Could you check a few things on this model? Use its own coordinates, in mm. A direction names the side the tool comes from. Coordinates: 2 decimals unless noted, no trailing zeros. Order: outer loops, then holes, each group sorted by start corner. A loop starts at its lowest first (then second) coordinate and runs counter-clockwise, first axis right, second up. Notation, with made-up numbers: (88, -19) -> (143, -19) arc R16 cw to (143, -10) -> close; hole circle Ø3 at (45, -25.5). An arc over 180 degrees is marked (long way). Use a Markdown table: item, result. Add a question column.
1) If we section it at C-C (y = 21): Write out the boundary of the cut face in (x, z), plus the area to 3 significant figures.
2) Will these pins go through, and if not, where does the flat tip stop? pin 1 Ø13 at (x, y) = (41.5, 57.5) entering from +Z; pin 2 Ø5 at (x, y) = (41.5, 57.5) entering from +Z; pin 3 Ø3 at (x, y) = (-41.5, 57.5) entering from +Z.
3) If we section it at B-B (y = -14.5): Write out the boundary of the cut face in (x, z).
4) If I drill on L1, parallel to Y at x = -41.5, z = 7.7; L2, parallel to X at y = 22, z = 1.75; L3, parallel to X at y = 32, z = 4, over which ranges is the centre line in solid material (lowest first)? Write a range as [from, to].
5) If we section it at A-A (x = 21.5): Write out the boundary of the cut face in (y, z).
6) Which directions (+Z, -Z, +X, -X, +Y, -Y) give clear straight access to the entire face, cutting with the end or side of a thin tool? Please do faces 5 (the flat face through (21.904, -4.523, 5.07)), 6 (the flat face through (-65, -2, 5)), 7 (the cylindrical face through (37.5, -28.5, 8)).
7) Thinking about a two-plate mould opening in Y: for faces 1 (the flat face through (-30.24, 46.57, 5.07)), 2 (the flat face through (14, 2, 0)), 3 (the cylindrical face through (-5.62, -26.266, 5.07)), 4 (the flat face through (-1, 120, 5)), which applies, +Y half, -Y half, draft (parallel to the pull), parting line (faces both ways), or undercut?
```python
from build123d import *

# Parameters (mm, degrees)
SKETCH008_W          = 130
SKETCH008_H          = 240
PAD005_DEPTH         = 10
SKETCH009_R          = 2
POCKET003_DEPTH      = 10.001
POCKET003_DEPTH_BACK = 0.001
SKETCH010_R          = 5
POCKET004_DEPTH      = 4
POCKET005_DEPTH      = 10.001
POCKET005_DEPTH_BACK = 0.001


with BuildPart() as part:
    # Sketch008 → Pad005 (new body)
    with BuildSketch(Plane.XY):
        Rectangle(SKETCH008_W, SKETCH008_H)
    extrude(amount=PAD005_DEPTH)

    # Sketch009 (on Face5 of Pad005) → Pocket003 (cut, two sides)
    with BuildSketch(Plane(origin=(0, 0, 0), x_dir=(1, 0, 0), z_dir=(0, 0, -1))) as pocket003_sk:
        with Locations((-41.5, -57.5)):
            Circle(SKETCH009_R)
        with Locations((-41.5, 25.5)):
            Circle(SKETCH009_R)
        with Locations((41.5, 25.5)):
            Circle(SKETCH009_R)
        with Locations((41.5, -57.5)):
            Circle(SKETCH009_R)
    extrude(amount=-POCKET003_DEPTH, mode=Mode.SUBTRACT)
    extrude(pocket003_sk.sketch, amount=POCKET003_DEPTH_BACK, mode=Mode.SUBTRACT)

    # Sketch010 (on Face5 of Pocket003) → Pocket004 (cut)
    with BuildSketch(Plane.XY.offset(10)):
        with Locations((-41.5, 57.5)):
            Circle(SKETCH010_R)
        with Locations((41.5, 57.5)):
            Circle(SKETCH010_R)
        with Locations((-41.5, -25.5)):
            Circle(SKETCH010_R)
        with Locations((41.5, -25.5)):
            Circle(SKETCH010_R)
    extrude(amount=-POCKET004_DEPTH, mode=Mode.SUBTRACT)

    # Sketch011 (on Face5 of Pocket004) → Pocket005 (cut, two sides)
    with BuildSketch(Plane.XY.offset(10)) as pocket005_sk:
        with BuildLine():
            ThreePointArc((-33.328427, -11.671573), (-33.328427, -17.328427), (-27.671573, -17.328427))
            Line((-27.671573, -17.328427), (33.328427, 43.671573))
            ThreePointArc((33.328427, 43.671573), (33.328427, 49.328427), (27.671573, 49.328427))
            Line((27.671573, 49.328427), (-33.328427, -11.671573))
        make_face()
        with BuildLine():
            ThreePointArc((-42.328427, -2.286797), (-42.328427, -7.943651), (-36.671573, -7.943651))
            Line((-36.671573, -7.943651), (23.943651, 52.671573))
            ThreePointArc((23.943651, 52.671573), (23.943651, 58.328427), (18.286797, 58.328427))
            Line((18.286797, 58.328427), (-42.328427, -2.286797))
        make_face()
        with BuildLine():
            ThreePointArc((-42.328427, 16.09798), (-42.328427, 10.441125), (-36.671573, 10.441125))
            Line((-36.671573, 10.441125), (5.558875, 52.671573))
            ThreePointArc((5.558875, 52.671573), (5.558875, 58.328427), (-0.09798, 58.328427))
            Line((-0.09798, 58.328427), (-42.328427, 16.09798))
        make_face()
        with BuildLine():
            ThreePointArc((-42.328427, 34.482756), (-42.328427, 28.825902), (-36.671573, 28.825902))
            Line((-36.671573, 28.825902), (-12.825902, 52.671573))
            ThreePointArc((-12.825902, 52.671573), (-12.825902, 58.328427), (-18.482756, 58.328427))
            Line((-18.482756, 58.328427), (-42.328427, 34.482756))
        make_face()
        with BuildLine():
            ThreePointArc((-23.943651, -20.671573), (-23.943651, -26.328427), (-18.286797, -26.328427))
            Line((-18.286797, -26.328427), (44.328427, 36.286797))
            ThreePointArc((44.328427, 36.286797), (44.328427, 41.943651), (38.671573, 41.943651))
            Line((38.671573, 41.943651), (-23.943651, -20.671573))
        make_face()
        with BuildLine():
            ThreePointArc((-5.558875, -20.671573), (-5.558875, -26.328427), (0.09798, -26.328427))
            Line((0.09798, -26.328427), (44.328427, 17.90202))
            ThreePointArc((44.328427, 17.90202), (44.328427, 23.558875), (38.671573, 23.558875))
            Line((38.671573, 23.558875), (-5.558875, -20.671573))
        make_face()
        with BuildLine():
            ThreePointArc((12.825902, -20.671573), (12.825902, -26.328427), (18.482756, -26.328427))
            Line((18.482756, -26.328427), (44.328427, -0.482756))
            ThreePointArc((44.328427, -0.482756), (44.328427, 5.174098), (38.671573, 5.174098))
            Line((38.671573, 5.174098), (12.825902, -20.671573))
        make_face()
    extrude(amount=-POCKET005_DEPTH, mode=Mode.SUBTRACT)
    extrude(pocket005_sk.sketch, amount=POCKET005_DEPTH_BACK, mode=Mode.SUBTRACT)


solid = part.part
```
Answer sheet:
| question | item | result |
|---|---|---|
| 1 | outline | (-65, 0) -> (-37.43, 0) -> (-37.43, 10) -> (-65, 10) -> close; (-26.11, 0) -> (-19.04, 0) -> (-19.04, 10) -> (-26.11, 10) -> close; (-7.73, 0) -> (-0.66, 0) -> (-0.66, 10) -> (-7.73, 10) -> close; (10.66, 0) -> (17.73, 0) -> (17.73, 10) -> (10.66, 10) -> close; (29.04, 0) -> (36.11, 0) -> (36.11, 10) -> (29.04, 10) -> close; (45.49, 0) -> (65, 0) -> (65, 10) -> (45.49, 10) -> close |
| 1 | area | 754 mm2 |
| 2 | pin 1 | z = 10 |
| 2 | pin 2 | z = 6 |
| 2 | pin 3 | through |
| 3 | outline | (-65, 0) -> (-34.5, 0) -> (-34.5, 10) -> (-65, 10) -> close; (-24.84, 0) -> (-17.77, 0) -> (-17.77, 10) -> (-24.84, 10) -> close; (-6.46, 0) -> (0.61, 0) -> (0.61, 10) -> (-6.46, 10) -> close; (11.93, 0) -> (19, 0) -> (19, 10) -> (11.93, 10) -> close; (30.31, 0) -> (65, 0) -> (65, 10) -> (30.31, 10) -> close |
| 4 | L1 | [-120, -30.5], [-20.5, -8.58], [-1.46, 9.81], [16.93, 28.19], [35.31, 52.5], [62.5, 120] |
| 4 | L2 | [-65, -36.43], [-25.11, -18.04], [-6.73, 0.34], [11.66, 18.73], [30.04, 37.11], [45.29, 65] |
| 4 | L3 | [-65, -43.49], [-33.5, -26.43], [-15.11, -8.04], [3.27, 10.34], [21.66, 28.73], [40.04, 65] |
| 5 | outline | (-120, 0) -> (-23.31, 0) -> (-23.31, 10) -> (-120, 10) -> close; (-12, 0) -> (-4.93, 0) -> (-4.93, 10) -> (-12, 10) -> close; (6.39, 0) -> (13.46, 0) -> (13.46, 10) -> (6.39, 10) -> close; (24.77, 0) -> (31.84, 0) -> (31.84, 10) -> (24.77, 10) -> close; (43.16, 0) -> (50.23, 0) -> (50.23, 10) -> (43.16, 10) -> close; (59.48, 0) -> (120, 0) -> (120, 10) -> (59.48, 10) -> close |
| 6 | face 5 | +Z, -Z |
| 6 | face 6 | +Z, -Z, -X, +Y, -Y |
| 6 | face 7 | +Z |
| 7 | face 1 | undercut |
| 7 | face 2 | draft |
| 7 | face 3 | undercut |
| 7 | face 4 | +Y half |
